Check sheet for the drawn part. Datum: minimum x, y, z corner. Units: mm. Round coordinates to 2 decimals unless told otherwise and drop trailing zeros. Write each loop counter-clockwise with the first axis right and the second up, starting at its lowest first coordinate (ties: lowest second). Pieces come first, ordered by that corner, then holes. Notation, with made-up numbers: (-12, -3) - (-6, -3) arc R16 ccw to (-6, 13) - close; hole circle Ø10 at (17.25, 89.25). An arc over 180 degrees is marked (long way). Answer as a JSON object with one key per item and string values.
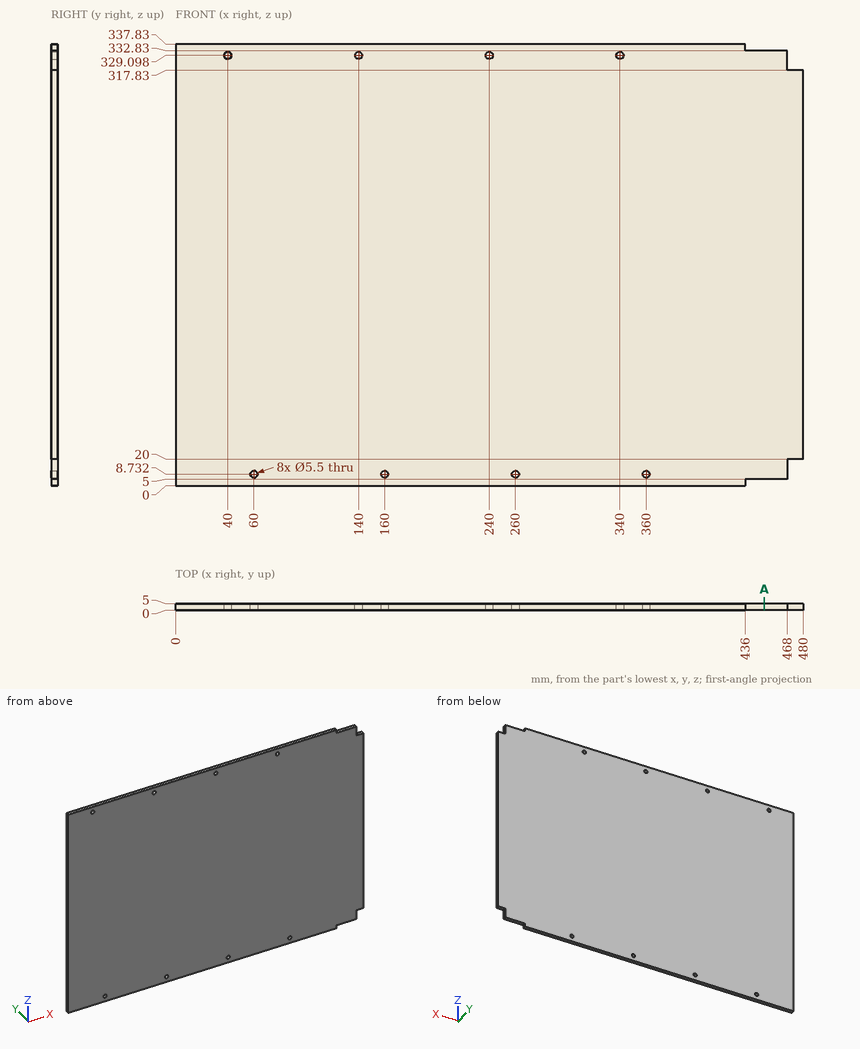
1. Cross-section at A-A (x = 450.5). Record the boundary of the cut face in (y, z).
Completed:
{"outline": "(0, 5) - (5, 5) - (5, 332.83) - (0, 332.83) - close"}
2. Material ranges on probe 1 along Z at (x, y) = (40, 3.65); probe 2 along Z at (x, y) = (160, 3.8), recorded low to high. Write a range as from..to.
Completed:
{"probe 1": "z = 0..326.35, 331.85..337.83", "probe 2": "z = 0..5.98, 11.48..337.83"}
3. Go/stop test with flat-tipped pins: pin 1 (3.5 mm diameter, centred on x = 240, z = 329.098, fed in from -Y); pin 2 (1.5 mm diameter, centred on y = 1.5, z = 12, fed in from +X); pin 3 (2.5 mm diameter, centred on x = 454, y = 3.5, fed in from +Z); pin 4 (1.5 mm diameter, centred on y = 3, z = 334.5, fed in from +X). Record where each tip stops, or that it passes through.
Completed:
{"pin 1": "passes through", "pin 2": "stops at x = 468", "pin 3": "stops at z = 332.83", "pin 4": "stops at x = 436"}
